Geometry check sheet. Reference: drawing and pictorial views, mm from the part's lowest x, y, z. Round coordinates to 2 decimals unless told otherwise and drop trailing zeros. Order: outer loops, then holes, each group sorted by start corner. A loop starts at its lowest first (then second) coordinate and runs counter-clockwise, first axis right, second up.
(1) Cross-section at A-A on z = 6.25. Enter the section's corners in (x, y) (1 decimal).
(2) Thickness scan on L1, parallel to Y at x = 5.25, z = 14.5 (1 decimal); L2, parallel to Z at x = 7.25, y = 2 (1 decimal); L3, parallel to X at y = 3, z = 1 (1 decimal). Record the ranges inside material, lowest first.
(3) Gauge pin test, flat ends, axial feed: P1, Ø2, axis at y = 6, z = 10, coming from the -X side; P2, Ø1.5, axis at x = 6, y = 5.5, coming from the +Z side. Record the tip position at first contact, or that the pin passes through.
(4) Cross-section at D-D on y = 5. Enter the section's corners in (x, z), and give its area (3 significant figures).
(5) Cross-section at B-B on y = 10.75. Enter the section's corners in (x, z), and give its area (3 significant figures).
(6) Cross-section at C-C on z = 9.5. Enter the section's corners in (x, y) (1 decimal).
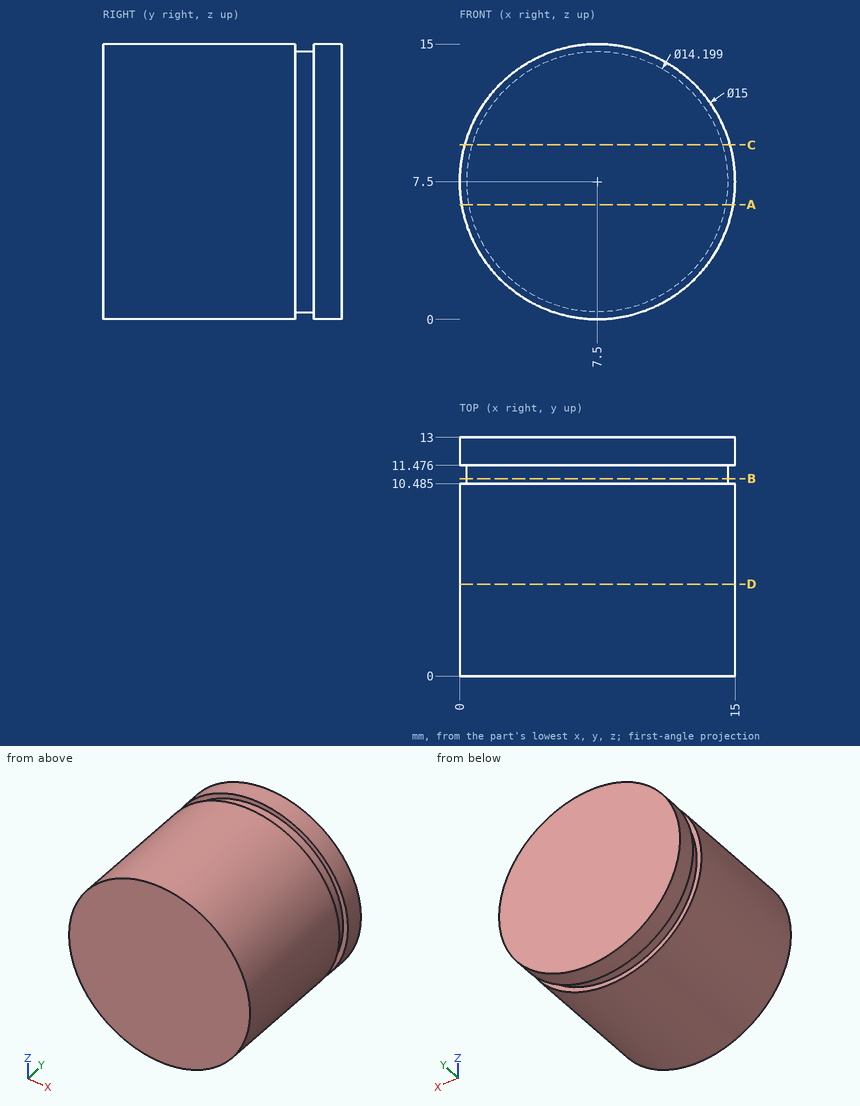
Found:
1. outline: (0.1, 0) - (14.9, 0) - (14.9, 10.5) - (14.5, 10.5) - (14.5, 11.5) - (14.9, 11.5) - (14.9, 13) - (0.1, 13) - (0.1, 11.5) - (0.5, 11.5) - (0.5, 10.5) - (0.1, 10.5) - close
2. L1: y = 0 to 10.5, 11.5 to 13
2. L2: z = 0 to 15
2. L3: x = 3.8 to 11.2
3. P1: stops at x = 0.15
3. P2: stops at z = 14.96
4. outline: circle Ø15 at (7.5, 7.5)
4. area: 177 mm2
5. outline: circle Ø14.2 at (7.5, 7.5)
5. area: 158 mm2
6. outline: (0.3, 0) - (14.7, 0) - (14.7, 10.5) - (14.3, 10.5) - (14.3, 11.5) - (14.7, 11.5) - (14.7, 13) - (0.3, 13) - (0.3, 11.5) - (0.7, 11.5) - (0.7, 10.5) - (0.3, 10.5) - close
